Could you check a few things on this model? Use its own coordinates, in mm. Face numbers are marked on the shaded views. A direction names the side the tool comes from. Coordinates: 2 decimals unless noted, no trailing zeros. Order: outer loops, then holes, each group sorted by start corner. A loop starts at its lowest first (then second) coordinate and runs counter-clockwise, first axis right, second up. Notation, with made-up numbers: (-24, 89) - (4, 89) arc R25 cw to (4, 110) - close; hole circle Ø8 at (58, 35.5). An arc over 180 degrees is marked (long way). Answer as CSV lines item,"result". Start each with the question number.
1. For pin 1 (1.5 mm diameter, centred on x = 57.5, z = 298, fed in from +Y); pin 2 (4 mm diameter, centred on y = 214.5, z = 332, fed in from +X) (3 decimals); pin 3 (10 mm diameter, centred on x = 39, y = 216, fed in from +Z); pin 4 (1 mm diameter, centred on y = 163, z = 82.5, fed in from +X), each with a flat end and sliding along its axis, tell me the tip position at first contact or that it passes through.
2. Thinking about a two-plate mould opening in X: for the marked faces 1, 2 and 3, which applies, released by +X, released by -X, zero draft, split by the parting line, or undercut?
3. I need wall thicknesses on probe 1 along Z at (x, y) = (-51, 188.5); probe 2 along X at (y, z) = (197, 361); probe 3 along X at (y, z) = (180.5, 499). Which ranges of each line are inside material? Lowest first, please.
4. For the marked faces 4 and 5, which set-ups out of +Z, -Z, +X, -X, +Y, -Y let a thin tool reach every point of the face, with its end or its side?
5. I want a section at A-A, the plane z = 87. List the corners of the cut face in (x, y) for me, and give its area (3 significant figures).
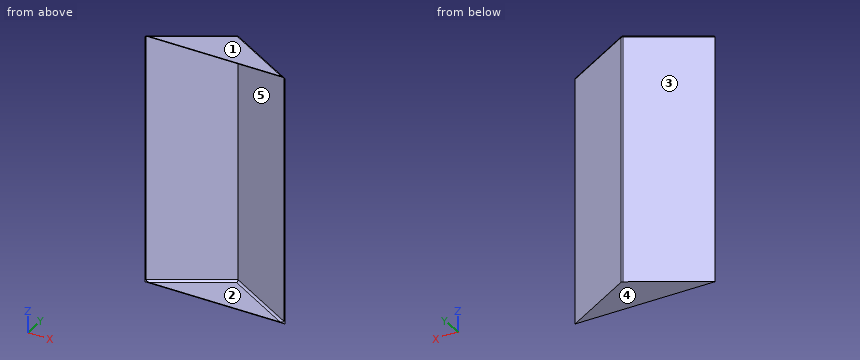
Autodesk Inventor part; units mm, degrees
ref_plane "YZ Plane" through (0, 0, 0) normal (1, 0, 0) x (0, 1, 0)
ref_plane "XZ Plane" through (0, 0, 0) normal (0, 1, 0) x (-1, 0, 0)
ref_plane "XY Plane" through (0, 0, 0) normal (0, 0, 1) x (1, 0, 0)
sketch "Boceto1" plane through (0, 0, 0) normal (0, 0, 1) x (1, 0, 0)
  line L0 (-146.2, 146.2) -> (146.2, 146.2)
  line L1 (-146.2, 146.2) -> (0, 230.6086)
  line L2 (-146.2, 146.2) -> (32.5033, 146.2) construction
  line L3 (0, 230.6086) -> (146.2, 146.2)
  point P0 (0, 0)
  dimension "d2" = 30
extrude "Extrusión1" add sketch "Boceto1" along normal blind 522.4
shell "Vaciado1" thickness 1.2 removed faces 1 at (-48.7333, 146.2, 174.1333)
fillet "Empalme1" radius 4 5 edges at (0, 230.6086, 261.2) (-73.1, 188.4043, 522.4) (73.1, 188.4043, 522.4) (71.9, 187.7115, 1.2) (-71.9, 187.7115, 1.2)
properties part number "tapa_marco"
Solved:
1,pin 1,"stops at y = 197.84"
1,pin 2,"stops at x = 31.365"
1,pin 3,"passes through"
1,pin 4,"stops at x = 117.97"
2,face 1,"zero draft"
2,face 2,"undercut"
2,face 3,"released by -X"
3,probe 1,"z = 0 to 1.2, 521.2 to 522.4"
3,probe 2,"x = -58.21 to -55.81, 55.81 to 58.21"
3,probe 3,"x = -86.79 to -84.39, 84.39 to 86.79"
4,face 4,"-Z, +X, -X, +Y, -Y"
4,face 5,"-Y"
5,outline,"(-146.2, 146.2) - (-143.8, 146.2) - (0, 229.22) - (143.8, 146.2) - (146.2, 146.2) - (2, 229.45) arc R4 ccw to (-2, 229.45) - close"
5,area,"401 mm2"
